Check sheet for the modelled part. Datum: model origin and axes. Units: mm. Face numbers are marked on the shaded views. A direction names the side the tool comes from. Give positions to 0.01 mm unless a question says otherwise; leave off trailing zeros. Order: outer loops, then holes, each group sorted by start corner. A loop starts at its lowest first (then second) coordinate and runs counter-clockwise, first axis right, second up. Notation, with made-up numbers: (-18, 13.5) -> (40, 13.5) arc R16 cw to (40, 42.5) -> close; hole circle Ø10 at (-4.75, 58). An arc over 180 degrees is marked (long way). Answer in a Markdown table with one row per item. Add a question column.
(1) Set-up check for the marked faces 1, 2 and 3: record each of +Z, -Z, +X, -X, +Y, -Y from which the full face is reachable in a straight line by a thin tool's end or side.
(2) Go/stop test with flat-tipped pins: pin 1 (8 mm diameter, centred on x = -9.25, y = 16.02, fed in from -Z); pin 2 (3 mm diameter, centred on x = 8.5, y = -15, fed in from +Z); pin 3 (19 mm diameter, centred on x = 1.5, y = -3.5, fed in from +Z). Record where each tip stops, or that it passes through.
(3) Thickness scan on L1, parallel to Y at x = 9.25, z = 2.65; L2, parallel to Y at x = -9.25, z = 5.75; L3, parallel to Y at x = -21.5, z = 8. Record the ranges inside material, lowest first. Write a range as [from, to].
(4) Cross-section at A-A (x = 0). Record the cut outline in (y, z), then the cut area to 4 significant figures.
(5) Cross-section at D-D (z = 8.25). Record the cut outline in (x, y).
(6) Cross-section at C-C (x = -9.25). Record the cut outline in (y, z).
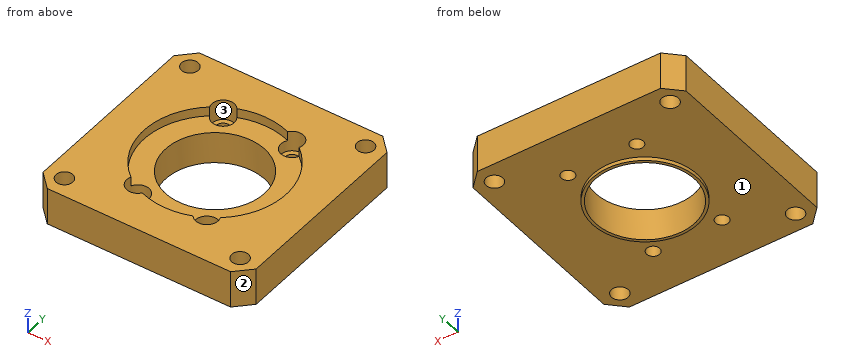
```python
from build123d import *

# Parameters (mm, degrees)
F0_W            = 57.2
F0_H            = 57.2
F1_DEPTH        = 10
F2_SIZE         = 4
F3_R            = 19.05
F4_DEPTH        = 2.5
F5_R            = 14
F6_DEPTH        = 1
F7_R            = 13.25
F8_DEPTH        = 8.501
F10_D           = 4.5
F12_D           = 3.5
F12_START       = 2.5
F12_CBORE_D     = 6
F12_CBORE_DEPTH = 3


with BuildPart() as f1:
    # F0 (on Top) → F1 (new body)
    with BuildSketch(Plane.XY):
        Rectangle(F0_W, F0_H)
    extrude(amount=F1_DEPTH)

    # F2
    f2_edges = [f1.edges().sort_by_distance(p)[0] for p in [
        (-28.6, 28.6, 5),
        (28.6, 28.6, 5),
        (28.6, -28.6, 5),
        (-28.6, -28.6, 5),
    ]]
    chamfer(f2_edges, length=F2_SIZE)

    # F3 (on face) → F4 (cut)
    with BuildSketch(Plane.XY.offset(10)):
        Circle(F3_R)
    extrude(amount=-F4_DEPTH, mode=Mode.SUBTRACT)

    # F5 (on face) → F6 (join)
    with BuildSketch(Plane(origin=(0, 0, 0), x_dir=(1, 0, 0), z_dir=(0, 0, -1))):
        Circle(F5_R)
    extrude(amount=F6_DEPTH)

    # F7 (on face) → F8 (cut, through all)
    with BuildSketch(Plane.XY.offset(7.5)):
        Circle(F7_R)
    extrude(amount=-F8_DEPTH, mode=Mode.SUBTRACT)

    # F10 (through all)
    with Locations(Plane.XY.offset(10)):
        with Locations((-23.5749400848, 23.5749400848), (23.5749400848, 23.5749400848), (23.5749400848, -23.5749400848), (-23.5749400848, -23.5749400848)):
            Hole(F10_D / 2)

    # F12 (through all)
    # its depths count from where the whole tool has entered the part; down to there all is cleared
    with Locations(Plane.XY.offset(10).offset(-F12_START)):
        with Locations((-9.25, 16.02146997), (9.25, 16.02146997), (9.25, -16.02146997), (-9.25, -16.02146997)):
            CounterBoreHole(F12_D / 2, F12_CBORE_D / 2, F12_CBORE_DEPTH)


solid = f1.part
```
Answer below:
| question | item | result |
|---|---|---|
| 1 | face 1 | -Z |
| 1 | face 2 | +Z, -Z, +X, -Y |
| 1 | face 3 | +Z |
| 2 | pin 1 | stops at z = 0 |
| 2 | pin 2 | stops at z = 4.5 |
| 2 | pin 3 | stops at z = 7.5 |
| 3 | L1 | y = [-28.6, -17.77], [-14.27, -9.49], [9.49, 14.27], [17.77, 28.6] |
| 3 | L2 | y = [-28.6, -19.02], [-13.02, -9.49], [9.49, 13.02], [19.02, 28.6] |
| 3 | L3 | y = [-28.6, -24.45], [-22.7, 22.7], [24.45, 28.6] |
| 4 | outline | (-28.6, 0) -> (-14, 0) -> (-14, -1) -> (-13.25, -1) -> (-13.25, 7.5) -> (-19.05, 7.5) -> (-19.05, 10) -> (-28.6, 10) -> close; (13.25, -1) -> (14, -1) -> (14, 0) -> (28.6, 0) -> (28.6, 10) -> (19.05, 10) -> (19.05, 7.5) -> (13.25, 7.5) -> close |
| 4 | area | 279.5 mm² |
| 5 | outline | (-28.6, -24.6) -> (-24.6, -28.6) -> (24.6, -28.6) -> (28.6, -24.6) -> (28.6, 24.6) -> (24.6, 28.6) -> (-24.6, 28.6) -> (-28.6, 24.6) -> close; hole circle Ø4.5 at (-23.57, -23.57); hole circle Ø4.5 at (-23.57, 23.57); hole (-11.99, -14.8) arc R3 ccw to (-6.82, -17.79) arc R19.05 ccw to (6.82, -17.79) arc R3 ccw to (11.99, -14.8) arc R19.05 ccw to (11.99, 14.8) arc R3 ccw to (6.82, 17.79) arc R19.05 ccw to (-6.82, 17.79) arc R3 ccw to (-11.99, 14.8) arc R19.05 ccw to start; hole circle Ø4.5 at (23.57, -23.57); hole circle Ø4.5 at (23.57, 23.57) |
| 6 | outline | (-28.6, 0) -> (-17.77, 0) -> (-17.77, 4.5) -> (-19.02, 4.5) -> (-19.02, 10) -> (-28.6, 10) -> close; (-14.27, 0) -> (-10.51, 0) -> (-10.51, -1) -> (-9.49, -1) -> (-9.49, 7.5) -> (-13.02, 7.5) -> (-13.02, 4.5) -> (-14.27, 4.5) -> close; (9.49, -1) -> (10.51, -1) -> (10.51, 0) -> (14.27, 0) -> (14.27, 4.5) -> (13.02, 4.5) -> (13.02, 7.5) -> (9.49, 7.5) -> close; (17.77, 0) -> (28.6, 0) -> (28.6, 10) -> (19.02, 10) -> (19.02, 4.5) -> (17.77, 4.5) -> close |
